CAD build for the part. Positions are in the model's coordinates, mm. Face numbers are marked on the shaded views. A direction names the side the tool comes from. Coordinates: 2 decimals unless noted, no trailing zeros. Loops run counter-clockwise (first coordinate to the right, second up) from the corner with the lowest first, then second, coordinate; pieces in that order, holes last. Notation, with made-up numbers: (17, 20.25) -> (59, 20.25) arc R33 cw to (59, 49.25) -> close; hole circle Ø7 at (12.5, 80). An arc over 180 degrees is marked (long way). Write each question's results on one line, items separated by ' | '.
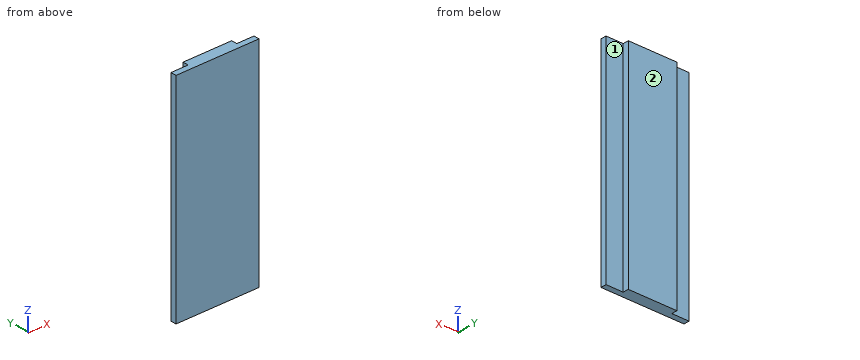
Autodesk Inventor part; units mm, degrees
ref_plane "YZ Plane" through (0, 0, 0) normal (1, 0, 0) x (0, 1, 0)
ref_plane "XZ Plane" through (0, 0, 0) normal (0, 1, 0) x (-1, 0, 0)
ref_plane "XY Plane" through (0, 0, 0) normal (0, 0, 1) x (1, 0, 0)
sketch "Sketch1" plane through (0, 0, 0) normal (0, 1, 0) x (-1, 0, 0)
  line L0 (20.0371, 36.1085) -> (-8.9629, 36.1085)
  line L1 (-8.9629, 36.1085) -> (-8.9629, -38.8915)
  line L2 (-8.9629, -38.8915) -> (20.0371, -38.8915)
  line L3 (20.0371, -38.8915) -> (20.0371, 36.1085)
  point P0 (0, 0)
  dimension "d0" = 75
  dimension "d1" = 29
extrude "Extrusion1" add sketch "Sketch1" along normal blind 2
sketch "Sketch2" plane through (0, 2, 0) normal (0, 1, 0) x (1, 0, 0)
  line L0 (-20.0371, -36.1085) -> (8.9629, -36.1085)
  line L1 (2.9629, -36.1085) -> (2.9629, 38.8915)
  line L2 (8.9629, 38.8915) -> (-20.0371, 38.8915)
  line L3 (-14.0371, -36.1085) -> (-14.0371, 38.8915)
  point P0 (0, 0)
  dimension "d4" = 6
  dimension "d5" = 6
extrude "Extrusion2" add sketch "Sketch2" along normal blind 2
Q1. Cut at B-B on y = 3. Write the cut outline in (x, z).
Results are:
outline: (-14.04, -38.89) -> (2.96, -38.89) -> (2.96, 36.11) -> (-14.04, 36.11) -> close
Q2. Drop flat-ended pins along their axis: pin 1 (1.8 mm diameter, centred on x = -17, z = -16, fed in from +Y); pin 2 (1.6 mm diameter, centred on y = 3.5, z = 12, fed in from -X). Give the stop position or say it passes through.
Results are:
pin 1: y = 2 | pin 2: x = -14.04
Q3. Wall check: L1, parallel to Y at x = 7.5, z = 13.5; L2, parallel to X at y = 2.9, z = -31. Give the ranges that are in metal, low to high. Write a range as from..to.
Results are:
L1: 0..2 | L2: -14.04..2.96
Q4. Which spindle directions (+Z, -Z, +X, -X, +Y, -Y) get a long thin tool onto all of the face, cutting with end or side? Do the marked faces 1 and 2. Say none if no direction does.
Results are:
face 1: +Z, -Z, +X, +Y | face 2: +Z, -Z, +X, -X, +Y
Q5. Cut at C-C on x = 7. Write the cut outline in (y, z).
Results are:
outline: (0, -38.89) -> (2, -38.89) -> (2, 36.11) -> (0, 36.11) -> close
Q6. Cut at A-A on z = -25.5. Write the cut outline in (x, y).
Results are:
outline: (-20.04, 0) -> (8.96, 0) -> (8.96, 2) -> (2.96, 2) -> (2.96, 4) -> (-14.04, 4) -> (-14.04, 2) -> (-20.04, 2) -> close
